Geometry: final body of the model. Coordinates: model frame, mm. Round coordinates to 2 decimals unless told otherwise and drop trailing zeros. Order: outer loops, then holes, each group sorted by start corner. A loop starts at its lowest first (then second) coordinate and runs counter-clockwise, first axis right, second up. Notation, with made-up numbers: (-24, 23.5) -> (12, 23.5) arc R26 cw to (12, 38.5) -> close; hole circle Ø3 at (62.25, -4). An arc over 180 degrees is marked (long way). Put each result on its own line as item: value.
```python
from build123d import *

# Parameters (mm, degrees)
SKETCH_1_W          = 17
SKETCH_1_H          = 21
EXTRUDE_1_DEPTH     = 1.6
SKETCH_2_W          = 2.4
SKETCH_2_H          = 6.4
CUT_EXTRUDE_1_DEPTH = 10
CUT_EXTRUDE_2_DEPTH = 10


with BuildPart() as part:
    # 草图1 → 凸台-拉伸1 (new body)
    with BuildSketch(Plane(origin=(0, 0, 0), x_dir=(1, 0, 0), z_dir=(0, 1, 0))):
        with Locations((-8.5, 10.5)):
            Rectangle(SKETCH_1_W, SKETCH_1_H)
    extrude(amount=EXTRUDE_1_DEPTH)

    # 草图2 → 切除-拉伸1 (cut)
    with BuildSketch(Plane(origin=(0, 1.6, 0), x_dir=(1, 0, 0), z_dir=(0, 1, 0))):
        with Locations((-8.5, 12.6)):
            Rectangle(SKETCH_2_W, SKETCH_2_H)
    extrude(amount=-CUT_EXTRUDE_1_DEPTH, mode=Mode.SUBTRACT)

    # 草图3 → 切除-拉伸2 (cut)
    with BuildSketch(Plane(origin=(0, 1.6, 0), x_dir=(1, 0, 0), z_dir=(0, 1, 0))):
        Polygon((0, 16.8), (-1.5, 16.8), (-2.1, 16.8), (-2.1, 15.6), (-1.5, 15.6), (-1.5, 9.2), (-2.1, 9.2), (-2.1, 8), (-1.5, 8), (0, 8), align=None)
    extrude(amount=-CUT_EXTRUDE_2_DEPTH, mode=Mode.SUBTRACT)


solid = part.part
```
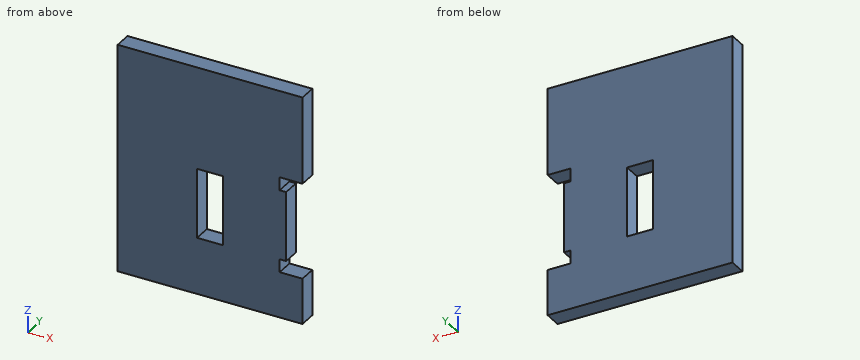
1. Material intervals for probe 1 along X at (y, z) = (0.8, -11.5); probe 2 along Z at (x, y) = (-1, 1.55); probe 3 along Z at (x, y) = (-9.25, 0.25), sorted ascending.
Ans:
probe 1: -17 to -9.7, -7.3 to -1.5
probe 2: -21 to -16.8, -8 to 0
probe 3: -21 to -15.8, -9.4 to 0
2. Cut plane C-C on y = 0.55. Return loops of the section in (x, z), and give its area (3 significant figures).
Ans:
outline: (-17, -21) -> (0, -21) -> (0, -16.8) -> (-2.1, -16.8) -> (-2.1, -15.6) -> (-1.5, -15.6) -> (-1.5, -9.2) -> (-2.1, -9.2) -> (-2.1, -8) -> (0, -8) -> (0, 0) -> (-17, 0) -> close; hole (-9.7, -15.8) -> (-7.3, -15.8) -> (-7.3, -9.4) -> (-9.7, -9.4) -> close
area: 327 mm²
3. Contact query for a flat-ended pin moving along its axis: P1, Ø0.5, axis at y = 1, z = -13, coming from the +X side. Output: stop coordinate, or through.
Ans:
P1: x = -1.5
4. Cut plane A-A on x = -8.75. Return loops of the section in (y, z).
Ans:
outline: (0, -21) -> (1.6, -21) -> (1.6, -15.8) -> (0, -15.8) -> close; (0, -9.4) -> (1.6, -9.4) -> (1.6, 0) -> (0, 0) -> close
5. Cut plane B-B on z = -11. Return loops of the section in (x, y), and give its area (3 significant figures).
Ans:
outline: (-17, 0) -> (-9.7, 0) -> (-9.7, 1.6) -> (-17, 1.6) -> close; (-7.3, 0) -> (-1.5, 0) -> (-1.5, 1.6) -> (-7.3, 1.6) -> close
area: 21.0 mm²
